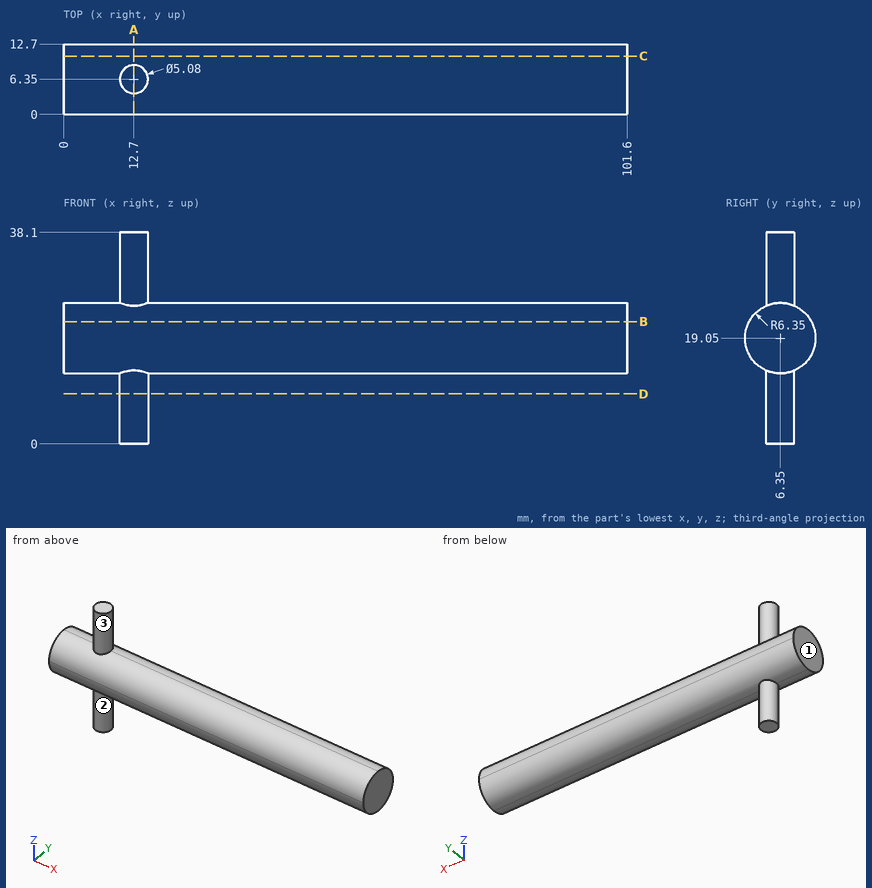
Job drawing, mm, ordinate dimensions from the low corner. One solid piece. A direction names the side the tool comes from. Coordinates: 2 decimals unless noted, no trailing zeros. Order: outer loops, then holes, each group sorted by start corner. A loop starts at its lowest first (then second) coordinate and runs counter-clockwise, first axis right, second up. Notation, with made-up numbers: (74.25, 9.5) -> (119.25, 9.5) arc R21 ccw to (119.25, 41.5) -> close; hole circle Ø9 at (89.25, 52). An arc over 180 degrees is marked (long way). Return JSON: item names as keys, results as strings. Group by question number.
Item 1: Saw through at C-C on y = 10.5. Write the cut outline in (x, z), then the cut area to 3 significant figures.
Item 2: Saw through at A-A on x = 12.7. Write the cut outline in (y, z), then the cut area to 3 significant figures.
Item 3: Saw through at D-D on z = 9. Write the cut outline in (x, y).
Item 4: Saw through at B-B on z = 22. Write the cut outline in (x, y), then the cut area to 3 significant figures.
Item 5: Flat gauge pins, fed straight in: P1, Ø3, axis at x = 53.5, y = 5, coming from the +Z side; P2, Ø6, axis at y = 5.5, z = 6, coming from the +X side; P3, Ø5, axis at x = 67.5, z = 25.5, coming from the +Y side. Where does each tip first touch, or does it go through?
Item 6: Wall check: line 1 along Z through (x, y) = (48, 6.25); line 2 along X through (y, z) = (7, 35.5); line 3 along Z through (x, y) = (72.5, 10.75). Give the ranges that are in metal, low to high. Write a range as [from, to].
Item 7: Tool access for the marked faces 1, 2 and 3: list every direction of +Z, -Z, +X, -X, +Y, -Y with a clear straight run to the whole face (end or side of a thin tool).
Values found:
{
 "1": {"outline": "(0, 14.24) -> (101.6, 14.24) -> (101.6, 23.86) -> (0, 23.86) -> close", "area": "977 mm2"},
 "2": {"outline": "(3.81, 0) -> (8.89, 0) -> (8.89, 13.23) arc R6.35 ccw to (8.89, 24.87) -> (8.89, 38.1) -> (3.81, 38.1) -> (3.81, 24.87) arc R6.35 ccw to (3.81, 13.23) -> close", "area": "257 mm2"},
 "3": {"outline": "circle Ø5.08 at (12.7, 6.35)"},
 "4": {"outline": "(0, 0.73) -> (101.6, 0.73) -> (101.6, 11.97) -> (0, 11.97) -> close", "area": "1,140 mm2"},
 "5": {"P1": "stops at z = 25.4", "P2": "stops at x = 15.24", "P3": "stops at y = 11.32"},
 "6": {"line 1": "z = [12.7, 25.4]", "line 2": "x = [10.24, 15.16]", "line 3": "z = [14.47, 23.63]"},
 "7": {"face 1": "+Z, -Z, -X, +Y, -Y", "face 2": "-Z", "face 3": "+Z"}
}
